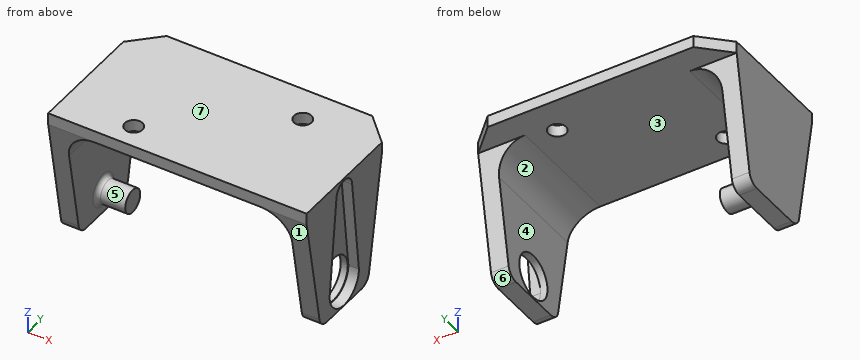
from build123d import *

# Parameters (mm, degrees)
SKETCH1_W           = 38
SKETCH1_H           = 20
BOSS_EXTRUDE1_DEPTH = 2
BOSS_EXTRUDE2_DEPTH = 3
BOSS_EXTRUDE3_DEPTH = 2
SKETCH4_R           = 1.6
CUT_EXTRUDE1_DEPTH  = 51.865017448
CUT_EXTRUDE2_START  = -1.2
CUT_EXTRUDE2_DEPTH  = 2
SKETCH6_R           = 3.75
CUT_EXTRUDE3_DEPTH  = 2.4
CUT_EXTRUDE4_DEPTH  = 34.693471178
SKETCH8_R           = 2
BOSS_EXTRUDE4_DEPTH = 8
FILLET1_R           = 0.8
FILLET2_R           = 5
SKETCH9_R           = 1.5
CUT_EXTRUDE5_DEPTH  = 10


with BuildPart() as part:
    # Sketch1 → Boss-Extrude1 (new body)
    with BuildSketch(Plane.XY):
        Rectangle(SKETCH1_W, SKETCH1_H)
    extrude(amount=BOSS_EXTRUDE1_DEPTH)

    # Sketch2 → Boss-Extrude2 (add)
    with BuildSketch(Plane(origin=(19, 0, 0), x_dir=(0, 0, -1), z_dir=(1, 0, 0))):
        with BuildLine():
            Line((-2, 10), (0, 10))
            Line((0, 10), (19.347296355, 6.588549649))
            ThreePointArc((19.347296355, 6.588549649), (20.532088886, 5.904509362), (21, 4.618934143))
            Line((21, 4.618934143), (21, -4.618934143))
            ThreePointArc((21, -4.618934143), (20.532088886, -5.904509362), (19.347296355, -6.588549649))
            Line((19.347296355, -6.588549649), (0, -10))
            Line((0, -10), (-2, -10))
            Line((-2, -10), (-2, 10))
        make_face()
    boss_extrude2 = extrude(amount=BOSS_EXTRUDE2_DEPTH)

    # Mirror1: Boss-Extrude2 across plane
    add(boss_extrude2.mirror(Plane(origin=(0, 0, 0), x_dir=(0, 0, 1), z_dir=(1, 0, 0))))

    # Sketch3 → Boss-Extrude3 (add)
    with BuildSketch(Plane(origin=(0, 0, 0), x_dir=(-1, 0, 0), z_dir=(0, 0, -1))):
        Polygon((-22, -10), (-17.5, -14.5), (17.5, -14.5), (22, -10), align=None)
        Polygon((-22, 10), (22, 10), (17.5, 14.5), (-17.5, 14.5), align=None)
    extrude(amount=-BOSS_EXTRUDE3_DEPTH)

    # Sketch4 → Cut-Extrude1 (cut, through all)
    with BuildSketch(Plane.ZY.offset(22)):
        with Locations((-17, 0)):
            Circle(SKETCH4_R)
    extrude(amount=-CUT_EXTRUDE1_DEPTH, mode=Mode.SUBTRACT)

    # Sketch5 → Cut-Extrude2 (cut)
    with BuildSketch(Plane.ZY.offset(-19).offset(CUT_EXTRUDE2_START)):
        with BuildLine():
            Line((-17, -3.9), (-0.5, -2.1))
            ThreePointArc((-0.5, -2.1), (1.6, 0), (-0.5, 2.1))
            Line((-0.5, 2.1), (-17, 3.9))
            ThreePointArc((-17, 3.9), (-20.9, 0), (-17, -3.9))
        make_face()
    extrude(amount=-CUT_EXTRUDE2_DEPTH, mode=Mode.SUBTRACT)

    # Sketch6 → Cut-Extrude3 (cut)
    with BuildSketch(Plane.ZY.offset(-19)):
        with Locations((-17, 0)):
            Circle(SKETCH6_R)
    extrude(amount=-CUT_EXTRUDE3_DEPTH, mode=Mode.SUBTRACT)

    # Sketch7 → Cut-Extrude4 (cut, through all)
    with BuildSketch(Plane(origin=(0, 0, 0), x_dir=(-1, 0, 0), z_dir=(0, 0, -1))):
        Polygon((17.5, -14.5), (22, -10), (19, -10), (-19, -10), (-22, -10), (-17.5, -14.5), align=None)
    extrude(amount=-CUT_EXTRUDE4_DEPTH, mode=Mode.SUBTRACT)

    # Sketch8 → Boss-Extrude4 (add)
    with BuildSketch(Plane.ZY.offset(22)):
        with Locations((-17, 0)):
            Circle(SKETCH8_R)
    extrude(amount=-BOSS_EXTRUDE4_DEPTH)

    # Fillet1
    fillet1_edges = [part.edges().sort_by_distance(p)[0] for p in [
        (-19, 0, -19),
    ]]
    fillet(fillet1_edges, radius=FILLET1_R)

    # Fillet2
    fillet2_edges = [part.edges().sort_by_distance(p)[0] for p in [
        (-19, 0, 0),
        (19, 0, 0),
    ]]
    fillet(fillet2_edges, radius=FILLET2_R)

    # Sketch9 → Cut-Extrude5 (cut)
    with BuildSketch(Plane(origin=(0, 0, 0), x_dir=(-1, 0, 0), z_dir=(0, 0, -1))):
        with Locations((-9.5, 8.5)):
            Circle(SKETCH9_R)
        with Locations((10, -6)):
            Circle(SKETCH9_R)
    extrude(amount=-CUT_EXTRUDE5_DEPTH, mode=Mode.SUBTRACT)


solid = part.part
The listing builds one solid part. Answer for the finished solid, in the listing's coordinates (mm). Face numbers are marked on the shaded views. A direction names the side the tool comes from. Coordinates: 2 decimals unless noted, no trailing zeros. Order: outer loops, then holes, each group sorted by start corner. A loop starts at its lowest first (then second) coordinate and runs counter-clockwise, first axis right, second up. Notation, with made-up numbers: (-4, 1.25) -> (53, 1.25) arc R25 ccw to (53, 30.25) -> close; hole circle Ø8 at (-9, 3.5). An arc over 180 degrees is marked (long way). Answer in a Markdown table with one row per item. Add a question column.
Item 1: Find the intervals of material crossed by L1, parallel to Y at x = -10, z = 0.7; L2, parallel to X at y = 4.25, z = -13; L3, parallel to X at y = 5.75, z = -4, in increasing order. Write a range as from..to.
Item 2: Find section A-A (y = 0). Write down the section's boundary in (x, z).
Item 3: Find section D-D (y = 8.5). Write down the section's boundary in (x, z), then the cut area to 3 significant figures.
Item 4: Each of these flat-tipped pins is pushed along its axis until it touches: P1, Ø7.5, axis at x = 4.5, y = 4, coming from the -Z side; P2, Ø4.5, axis at y = -1, z = -17.5, coming from the +X side. Where does it stop, or does it pass through?
Item 5: Determine the mould class of the marked faces 4, 5, 6 and 7 for opening direction Z: +Z half, -Z half, draft (parallel to the pull), parting line (faces both ways), or undercut.
Item 6: Which of the six approach directions +Z, -Z, +X, -X, +Y, -Y give full straight-line access (tool end or side, diameter ignored) to the marked faces 1, 2 and 3?
Item 7: Find section B-B (x = 9.5). Write down the section's boundary in (y, z), then the cut area to 3 significant figures.
Item 8: Find section C-C (z = -11.5). Write down the section's boundary in (x, y), then the cut area to 3 significant figures.
Result set:
| question | item | result |
|---|---|---|
| 1 | L1 | y = -10..-7.5, -4.5..14.5 |
| 1 | L2 | x = -22..-19, 19..22 |
| 1 | L3 | x = -22..-18.9, 18.9..22 |
| 2 | outline | (-22, -21) -> (-19, -21) -> (-19, -19.8) arc R0.8 cw to (-18.2, -19) -> (-14, -19) -> (-14, -15) -> (-18.2, -15) arc R0.8 cw to (-19, -14.2) -> (-19, -5) arc R5 cw to (-14, 0) -> (14, 0) arc R5 cw to (19, -5) -> (19, -13.25) -> (20.2, -13.25) -> (20.2, 1.6) -> (22, 1.6) -> (22, 2) -> (-22, 2) -> close; (19, -21) -> (22, -21) -> (22, -20.9) -> (20.2, -20.9) -> (20.2, -20.75) -> (19, -20.75) -> close |
| 3 | outline | (-22, -8.51) -> (-19, -8.51) -> (-19, -5) arc R5 cw to (-14, 0) -> (8, 0) -> (8, 2) -> (-22, 2) -> close; (11, 0) -> (14, 0) arc R5 cw to (19, -5) -> (19, -8.51) -> (22, -8.51) -> (22, 2) -> (11, 2) -> close |
| 3 | area | 144 mm² |
| 4 | P1 | stops at z = 0 |
| 4 | P2 | stops at x = -14 |
| 5 | face 4 | draft |
| 5 | face 5 | undercut |
| 5 | face 6 | -Z half |
| 5 | face 7 | +Z half |
| 6 | face 1 | -Z, +X, -X, -Y |
| 6 | face 2 | -Z, +Y, -Y |
| 6 | face 3 | -Z, +Y |
| 7 | outline | (-10, 0) -> (7, 0) -> (7, 2) -> (-10, 2) -> close; (10, 0) -> (14.5, 0) -> (14.5, 2) -> (10, 2) -> close |
| 7 | area | 43.0 mm² |
| 8 | outline | (-22, -7.97) -> (-19, -7.97) -> (-19, 7.97) -> (-22, 7.97) -> close; (19, -7.97) -> (22, -7.97) -> (22, -3.3) -> (20.2, -3.3) -> (20.2, 3.3) -> (22, 3.3) -> (22, 7.97) -> (19, 7.97) -> close |
| 8 | area | 83.8 mm² |
